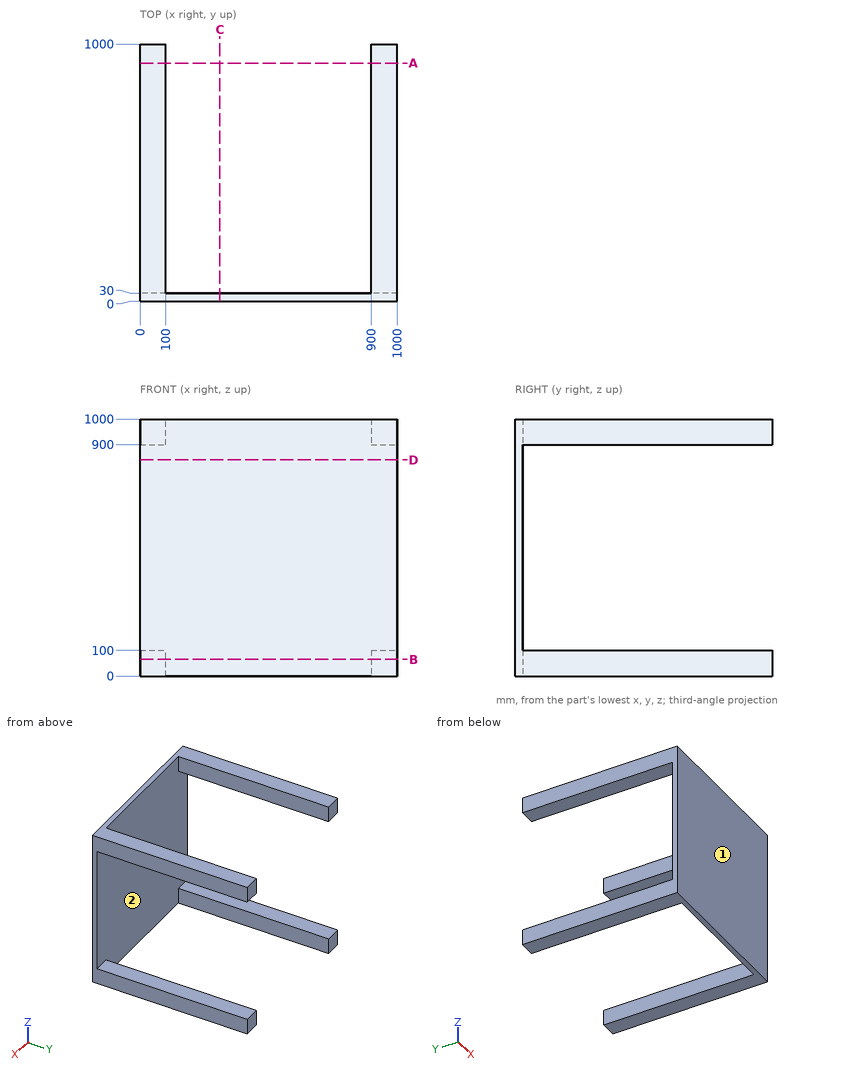
Design review of the part shown in the three views and the two pictorial views. Dimensions are in mm from the part's minimum x, y and z. Coordinates: 2 decimals unless noted, no trailing zeros. Loops run counter-clockwise (first coordinate to the right, second up) from the corner with the lowest first, then second, coordinate; pieces in that order, holes last.
Q1. The part is to be moulded in two halves that separate along X. For the marked faces 1 and 2, say which applies: +X half, -X half, draft (parallel to the pull), parting line (faces both ways), or undercut.
Reported:
face 1: draft
face 2: undercut
Q2. We need section B-B on z = 65. State the section outline as (x, y) points, and give its area (3 significant figures).
Reported:
outline: (0, 0) - (1000, 0) - (1000, 1000) - (900, 1000) - (900, 30) - (100, 30) - (100, 1000) - (0, 1000) - close
area: 224,000 mm2
Q3. We need section D-D on z = 841. State the section outline as (x, y) points, and give its area (3 significant figures).
Reported:
outline: (0, 0) - (1000, 0) - (1000, 30) - (0, 30) - close
area: 30,000 mm2
Q4. For pin 1 (2 mm diameter, centred on x = 751.5, z = 451, fed in from +Y), flat-tipped, find the tip position at first contact; note if it passes through.
Reported:
pin 1: stops at y = 30
Q5. To check wall thickness, follow line 1 (Z direction, x = 77, y = 568); line 2 (Y direction, x = 916, z = 138.5). State the ranges of each line that lie inside material, in increasing order.
Reported:
line 1: z = 0 to 100, 900 to 1000
line 2: y = 0 to 30
Q6. We need section A-A on y = 926. State the section outline as (x, z) points.
Reported:
outline: (0, 0) - (100, 0) - (100, 100) - (0, 100) - close; (0, 900) - (100, 900) - (100, 1000) - (0, 1000) - close; (900, 0) - (1000, 0) - (1000, 100) - (900, 100) - close; (900, 900) - (1000, 900) - (1000, 1000) - (900, 1000) - close
Q7. We need section C-C on x = 311. State the section outline as (y, z) points, and give its area (3 significant figures).
Reported:
outline: (0, 0) - (30, 0) - (30, 1000) - (0, 1000) - close
area: 30,000 mm2
